Here's how the part is built. I have some questions about the finished solid (model axes, mm). Face numbers are marked on the shaded views. A direction names the side the tool comes from. Coordinates: 2 decimals unless noted, no trailing zeros. Order: outer loops, then holes, each group sorted by start corner. A loop starts at its lowest first (then second) coordinate and runs counter-clockwise, first axis right, second up. Notation, with made-up numbers: (51.5, 9.25) - (83.5, 9.25) arc R21 cw to (83.5, 43.25) - close; hole circle Ø3 at (44.25, 89.5). An arc over 180 degrees is marked (long way). Answer as CSV lines item,"result". Start each with the question number.
Q1. Suppose I cut it at C-C (z = 17). Please give me the cut outline in (x, y), then the cut area to 3 significant figures.
Q2. For the marked faces 4, 5 and 6, which set-ups out of +Z, -Z, +X, -X, +Y, -Y let a thin tool reach every point of the face, with its end or its side?
Q3. Suppose I cut it at B-B (y = -1). Please give me the cut outline in (x, z).
Q4. I need wall thicknesses on line 1 (X direction, y = -4, z = 5); line 2 (X direction, y = -0.25, z = -2); line 3 (Z direction, x = -4.75, y = -1.75). Which ranges of each line are inside material? Lowest first, please.
Q5. For pin 1 Ø3 at (x, y) = (9, -6) entering from +Z; pin 2 Ø5 at (y, z) = (-7.5, 15.5) entering from +X; pin 3 Ø3 at (x, y) = (-5.5, -5.5) entering from -Z, each with a flat end and sliding along its axis, tell me the tip position at first contact or that it passes through.
Q6. Suppose I cut it at A-A (z = 0). Please give me the cut outline in (x, y), then the cut area to 3 significant figures.
Q7. Thinking about a two-plate mould opening in Z: for the marked faces 1, 2 and 3, which applies, released by +Z, released by -Z, zero draft, split by the parting line, or undercut?
from build123d import *

# Parameters (mm, degrees)
F0_R     = 3.65
F1_DEPTH = 10
F2_R     = 5
F3_SIZE  = 1


with BuildPart() as f1:
    # F0 (on Front) → F1 (new body)
    with BuildSketch(Plane.XZ):
        with BuildLine():
            Line((-1.5, 32), (-1.5, 5.964269))
            ThreePointArc((-1.5, 5.964269), (0, -6.15), (1.5, 5.964269))
            Line((1.5, 5.964269), (1.5, 32))
            Line((1.5, 32), (1.5, 33.995855))
            ThreePointArc((1.5, 33.995855), (6.49123, 33.437665), (11.349069, 32.162768))
            Line((11.349069, 32.162768), (11.922919, 35.134547))
            ThreePointArc((11.922919, 35.134547), (-0.341827, 37.018449), (-12.551888, 34.807689))
            Line((-12.551888, 34.807689), (-11.028524, 32.162768))
            ThreePointArc((-11.028524, 32.162768), (-6.328333, 33.407946), (-1.5, 33.981945))
            Line((-1.5, 33.981945), (-1.5, 32))
        make_face()
        Circle(F0_R, mode=Mode.SUBTRACT)
    extrude(amount=F1_DEPTH)

    # F2
    f2_edges = [f1.edges().sort_by_distance(p)[0] for p in [
        (1.5, -5, 33.995855),
        (-1.5, -5, 33.981945),
        (1.5, -5, 5.964269),
        (-1.5, -5, 5.964269),
    ]]
    fillet(f2_edges, radius=F2_R)

    # F3
    f3_edges = [f1.edges().sort_by_distance(p)[0] for p in [
        (-1.5, -10, 18.661073),
        (-2.051742, -10, 6.776187),
        (-3.387544, -10, 32.175892),
        (0, -10, -6.15),
        (-9.33922, -10, 32.692204),
        (2.051742, -10, 6.776187),
        (-11.790206, -10, 33.485228),
        (1.5, -10, 18.697149),
        (-0.341827, -10, 37.018449),
        (3.365873, -10, 32.23071),
        (11.635994, -10, 33.648657),
        (9.474964, -10, 32.744415),
        (-3.65, -10, 0),
    ]]
    chamfer(f3_edges, length=F3_SIZE)


solid = f1.part
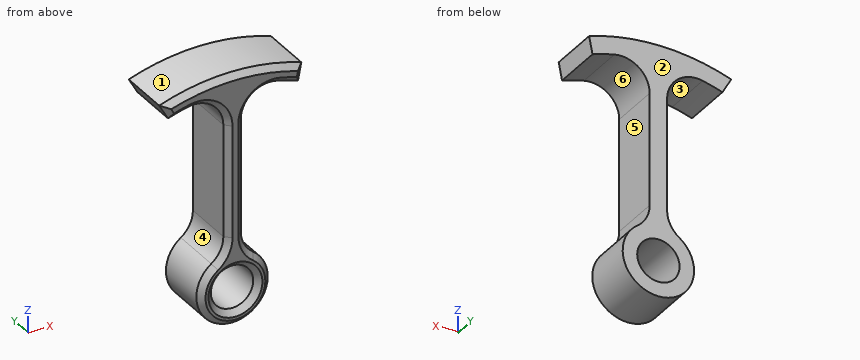
Here are the results:
1,outline,"(-1.5, -9) - (-0.5, -10) - (0.5, -10) - (1.5, -9) - (1.5, 0) - (-1.5, 0) - close"
1,area,"29.0 mm²"
2,face 4,"-X, +Y, -Y"
2,face 5,"+X, +Y, -Y"
2,face 6,"+Y, -Y"
3,outline,"(-12.55, 34.81) - (-11.03, 32.16) arc R34.6 cw to (-7.63, 33.13) arc R5 cw to (-1.5, 28.26) - (-1.5, 9.06) arc R5 cw to (-3.59, 5) arc R6.15 ccw (long way) to (3.59, 5) arc R5 cw to (1.5, 9.06) - (1.5, 28.33) arc R5 cw to (7.57, 33.22) arc R34.6 cw to (11.35, 32.16) - (11.92, 35.13) arc R37.6 ccw to start; hole circle Ø7.3 at (0, 0)"
4,line 1,"x = -3.58 to 3.58"
4,line 2,"x = -5.82 to -3.05, 3.05 to 5.82"
4,line 3,"z = -3.91 to 3.91, 32.95 to 36.7"
5,pin 1,"stops at z = 36.3"
5,pin 2,"stops at x = 1.5"
5,pin 3,"stops at z = -4.67"
6,outline,"(-6.15, -9) - (-5.15, -10) - (-4.65, -10) - (-3.65, -9) - (-3.65, 0) - (-6.15, 0) - close; (3.65, -9) - (4.65, -10) - (5.15, -10) - (6.15, -9) - (6.15, 0) - (3.65, 0) - close"
6,area,"48.0 mm²"
7,face 1,"released by +Z"
7,face 2,"zero draft"
7,face 3,"undercut"
